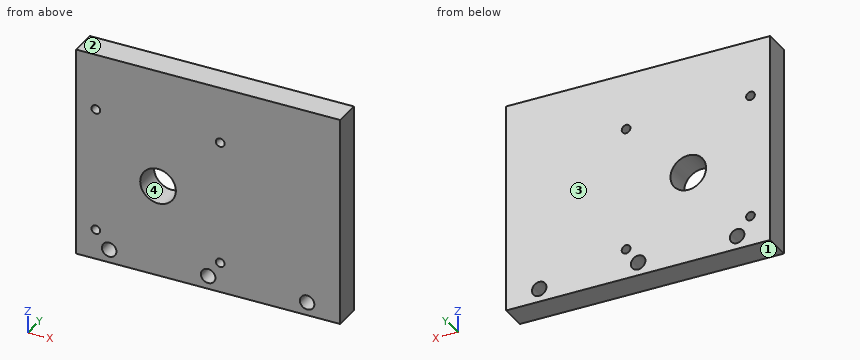
from build123d import *

# Parameters (mm, degrees)
F0_W     = 100
F0_H     = 80
F1_DEPTH = 10
F3_D     = 3.3
F4_D     = 13.5
F5_D     = 5.5
F5_DEPTH = 14.4
F5_TIP   = 1.6523667023


with BuildPart() as f1:
    # F0 (on Front) → F1 (new body)
    with BuildSketch(Plane.XZ):
        Rectangle(F0_W, F0_H)
    extrude(amount=F1_DEPTH)

    # F3 (through all)
    with Locations(Plane.XZ.offset(10)):
        with Locations((-42.57, 18.57), (4.57, 18.57), (-42.57, -28.57), (4.57, -28.57)):
            Hole(F3_D / 2)

    # F4 (through all)
    with Locations(Plane.XZ.offset(10)):
        with Locations((-19, -5)):
            Hole(F4_D / 2)

    # F5
    with Locations(Plane.XZ.offset(10)):
        with Locations((-37.5, -35), (0, -35), (37.5, -35)):
            Hole(F5_D / 2, depth=F5_DEPTH)
            with Locations((0, 0, -(F5_DEPTH + F5_TIP / 2))):  # 118° drill point
                Cone(0, F5_D / 2, F5_TIP, mode=Mode.SUBTRACT)


solid = f1.part
For this review, take the finished solid that the model builds, in its own axes (mm). Face numbers are marked on the shaded views. Round coordinates to 2 decimals unless told otherwise and drop trailing zeros. Write each loop counter-clockwise with the first axis right and the second up, starting at its lowest first coordinate (ties: lowest second). Pieces come first, ordered by that corner, then holes. Notation, with made-up numbers: (41, 88.5) - (45, 88.5) arc R24 cw to (45, 113.5) - close; hole circle Ø10 at (41.25, 5.5). An arc over 180 degrees is marked (long way). Write item = value, one per line. Start each with the question number.
1. Consider section D-D on x = 4.57. State the section outline as (y, z) points, plus the area to 3 significant figures.
2. Wall thickness on L1, parallel to Z at x = 4.57, y = -3.25; L2, parallel to Z at x = -19, y = -3.75; L3, parallel to Z at x = -37.5, y = -2.25: over which ranges is each line inside the solid? List them lowest first.
3. Consider section C-C on y = -7.5. Give the number of separate pieces and of enclosed holes in the cut face, plus the area to 3 significant figures.
4. For pin 1 Ø7 at (x, z) = (0, -35) entering from +Y, flat-tipped, find the tip position at first contact; note if it passes through.
5. Consider section B-B on x = -37.5. State the section outline as (y, z) points.
6. Consider section A-A on z = -28.57. State the section outline as (x, y) points, plus the area to 3 significant figures.
7. Draft analysis for pull direction Z (two halves, no side actions). For the marked faces 1, 2, 3 and 4, state which applies: released by +Z, released by -Z, zero draft, split by the parting line, or undercut.
Evaluation:
q1.outline = (-10, -40) - (0, -40) - (0, -30.22) - (-10, -30.22) - close; (-10, -26.92) - (0, -26.92) - (0, 16.92) - (-10, 16.92) - close; (-10, 20.22) - (0, 20.22) - (0, 40) - (-10, 40) - close
q1.area = 734 mm2
q2.L1 = -40 to -30.22, -26.92 to 16.92, 20.22 to 40
q2.L2 = -40 to -11.75, 1.75 to 40
q2.L3 = -40 to -37.75, -32.25 to 40
q3.separate_pieces = 1
q3.enclosed_holes = 8
q3.area = 7,750 mm2
q4.pin_1 = 0
q5.outline = (-10, -40) - (0, -40) - (0, -37.75) - (-10, -37.75) - close; (-10, -32.25) - (0, -32.25) - (0, 40) - (-10, 40) - close
q6.outline = (-50, -10) - (-44.22, -10) - (-44.22, 0) - (-50, 0) - close; (-40.92, -10) - (2.92, -10) - (2.92, 0) - (-40.92, 0) - close; (6.22, -10) - (50, -10) - (50, 0) - (6.22, 0) - close
q6.area = 934 mm2
q7.face_1 = released by -Z
q7.face_2 = released by +Z
q7.face_3 = zero draft
q7.face_4 = undercut
